```python
from build123d import *

# Parameters (mm, degrees)
ESQUISSE1_R        = 5
BOSS_EXTRU_1_DEPTH = 5
ESQUISSE6_R        = 35
ESQUISSE6_R_2      = 30
BOSS_EXTRU_6_DEPTH = 5
BOSS_EXTRU_9_DEPTH = 30
CONG_3_R           = 5


with BuildPart() as part:
    # Esquisse1 → Boss.-Extru.1 (new body)
    with BuildSketch(Plane.XY):
        with BuildLine():
            Line((-45.620718977, 15), (-70, 15))
            Line((-70, 15), (-70, -15))
            Line((-70, -15), (-45.620718977, -15))
            ThreePointArc((-45.620718977, -15), (-36.774201608, -17.062911874), (-29.752642811, -22.826086957))
            ThreePointArc((-29.752642811, -22.826086957), (37.5, 0), (-29.752642811, 22.826086957))
            ThreePointArc((-29.752642811, 22.826086957), (-36.774201608, 17.062911874), (-45.620718977, 15))
        make_face()
        Circle(ESQUISSE1_R, mode=Mode.SUBTRACT)
    extrude(amount=BOSS_EXTRU_1_DEPTH)

    # Esquisse6 → Boss.-Extru.6 (add)
    with BuildSketch(Plane.XY.offset(5)):
        Circle(ESQUISSE6_R)
        Circle(ESQUISSE6_R_2, mode=Mode.SUBTRACT)
    extrude(amount=BOSS_EXTRU_6_DEPTH)

    # Esquisse8 → Boss.-Extru.9 (add)
    with BuildSketch(Plane.XY.offset(5)):
        with BuildLine():
            Line((-70, -15), (-70, 15))
            Line((-70, 15), (-43.874821937, 15))
            ThreePointArc((-43.874821937, 15), (-39.966142137, 13.118047822), (-38.999841722, 8.888888889))
            ThreePointArc((-38.999841722, 8.888888889), (-40, 0), (-38.999841722, -8.888888889))
            ThreePointArc((-38.999841722, -8.888888889), (-39.966142137, -13.118047822), (-43.874821937, -15))
            Line((-43.874821937, -15), (-70, -15))
        make_face()
    extrude(amount=BOSS_EXTRU_9_DEPTH)

    # Congé3
    cong_3_edges = [part.edges().sort_by_distance(p)[0] for p in [
        (37.5, 0, 0),
        (-57.810359489, 15, 0),
        (-57.810359489, -15, 0),
        (-36.774201608, -17.062911874, 0),
        (-36.774201608, 17.062911874, 0),
    ]]
    fillet(cong_3_edges, radius=CONG_3_R - 0.0001)  # a hair under: the kernel refuses the full size


solid = part.part
```
Source: CAD feature listing. Evaluate the final solid. Frame: model axes, mm. A direction names the side the tool comes from. Give positions to 0.01 mm unless a question says otherwise; leave off trailing zeros. Loops run counter-clockwise (first coordinate to the right, second up) from the corner with the lowest first, then second, coordinate; pieces in that order, holes last. Notation, with made-up numbers: M 49.5,-3.75 L 107.5,-3.75 A32 ccw 107.5,25.25 Z; hole C -29.5,-1.5 d8. An arc over 180 degrees is marked long. Put each result on its own line as item: value.
Q1. Section D-D (z = 29). Return the cut outline in (x, y), and give its area (3 significant figures).
Response values:
outline: M -70,-15 L -43.87,-15 A5 ccw -39,-8.89 A40 cw -39,8.89 A5 ccw -43.87,15 L -70,15 Z
area: 909 mm²
Q2. Section C-C (x = -60.5). Return the cut outline in (y, z).
Response values:
outline: M -15,5 A5 ccw -10,0 L 10,0 A5 ccw 15,5 L 15,35 L -15,35 Z
Q3. Mould query, pull axis X, two halves, no side actions, for faces 4 (the cylindrical face through (-29.97, 1.32, 7.46)), 5 (the flat face through (-70, 0, 17)), 6 (the cylindrical face through (-58, -14, 2)). Classes: released by +X, released by -X, zero draft, split by the parting line, or undercut.
Response values:
face 4: undercut
face 5: released by -X
face 6: zero draft
Q4. Section A-A (z = 6.5). Return the cut outline in (x, y), and give its area (3 significant figures).
Response values:
outline: M -70,-15 L -43.87,-15 A5 ccw -39,-8.89 A40 cw -39,8.89 A5 ccw -43.87,15 L -70,15 Z; C 0,0 d70; hole C 0,0 d60
area: 1,930 mm²
Q5. Reachability of faces 1 (the flat face through (-57, 15, 20)), 2 (the cylindrical face through (-40, 0, 20)), 3 (the flat face through (26, 16, 10)) from +Z, -Z, +X, -X, +Y, -Y: full face, straight path, thin tool, end or side. Return the list, or none.
Response values:
face 1: +Z, -Z, -X, +Y
face 2: +Z
face 3: +Z, +X, +Y, -Y
Q6. Pin query (flat end, axial travel): P1, Ø8, axis at x = -50.5, y = 18.5, coming from the -Z side; P2, Ø5, axis at x = -38, z = 31.5, coming from the +Y side; P3, Ø21, axis at x = -55.5, z = 14.5, coming from the +Y side. Return the tip coordinate at first contact, or that it passes through.
Response values:
P1: stops at z = 2.82
P2: stops at y = 13.69
P3: stops at y = 15
Q7. Line query: probe 1 along X at (y, z) = (1.5, 7); probe 2 along Z at (x, y) = (23.5, -7); probe 3 along X at (y, z) = (9, 13). Output: solid intervals per line, ascending. Write a range as [from, to].
Response values:
probe 1: x = [-70, -39.97], [-34.97, -29.96], [29.96, 34.97]
probe 2: z = [0, 5]
probe 3: x = [-70, -38.98]
